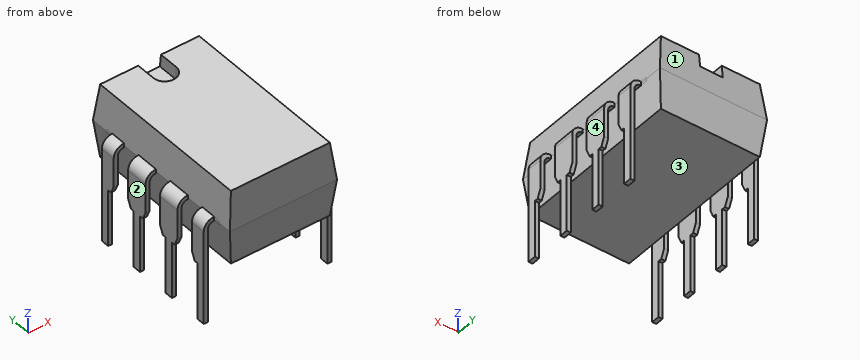
```python
from build123d import *

# Parameters (mm, degrees)
BASIC_SHAPE_DEPTH              = 5.46
SIDE_PROFILE1_DEPTH            = 4.3
SIDE_PROFILE1_DEPTH_BACK       = 4.3
SIDE_PROFILE2_DEPTH            = 4.3
SIDE_PROFILE2_DEPTH_BACK       = 4.3
LOCATION_MARK_DEPTH            = 0.8
SKETCH6_W                      = 0.25
SKETCH6_H                      = 1.39
PIN_RELIEF_DEPTH               = 8.235
REMAINING_PINS_COUNT           = 4
REMAINING_PINS_PITCH           = 2.54
REMAINING_PINS_COPY_1_SKETCH_W = 0.25
REMAINING_PINS_COPY_1_SKETCH_H = 1.39
REMAINING_PINS_COPY_2_SKETCH_W = 0.25
REMAINING_PINS_COPY_2_SKETCH_H = 1.39
REMAINING_PINS_COPY_3_SKETCH_W = 0.25
REMAINING_PINS_COPY_3_SKETCH_H = 1.39
REMAINING_PINS_COPY_4_DEPTH    = 8.235
REMAINING_PINS_COPY_5_DEPTH    = 8.235
REMAINING_PINS_COPY_6_DEPTH    = 8.235
PIN_SHAPE1_DEPTH               = 0.445
PIN_SHAPE2_DEPTH               = 0.445


with BuildPart() as part:
    # Sketch1 → Basic Shape (new body, symmetric)
    with BuildSketch(Plane(origin=(0, 0, 0), x_dir=(1, 0, 0), z_dir=(0, 1, 0))):
        Polygon((-3.05, -0.51), (-3.3, -2.795), (-3.05, -5.08), (3.05, -5.08), (3.3, -2.795), (3.05, -0.51), align=None)
    extrude(amount=BASIC_SHAPE_DEPTH, both=True)

    # Sketch2 → Side Profile1 (cut, two sides)
    with BuildSketch(Plane(origin=(0, 0, 0), x_dir=(0, 0, -1), z_dir=(1, 0, 0))) as side_profile1_sk:
        Polygon((-5.08, 5.46), (-5.08, 5.21), (-2.795, 5.46), align=None)
        Polygon((-5.08, -5.46), (-2.795, -5.46), (-5.08, -5.21), align=None)
    extrude(amount=SIDE_PROFILE1_DEPTH, mode=Mode.SUBTRACT)
    extrude(side_profile1_sk.sketch, amount=-SIDE_PROFILE1_DEPTH_BACK, mode=Mode.SUBTRACT)

    # Sketch3 → Side Profile2 (cut, two sides)
    with BuildSketch(Plane(origin=(0, 0, 0), x_dir=(0, 0, -1), z_dir=(1, 0, 0))) as side_profile2_sk:
        Polygon((-2.795, 5.46), (-0.51, 5.46), (-0.51, 5.21), align=None)
        Polygon((-2.795, -5.46), (-0.51, -5.46), (-0.51, -5.21), align=None)
    extrude(amount=SIDE_PROFILE2_DEPTH, mode=Mode.SUBTRACT)
    extrude(side_profile2_sk.sketch, amount=-SIDE_PROFILE2_DEPTH_BACK, mode=Mode.SUBTRACT)

    # Sketch4 → Location Mark (cut)
    with BuildSketch(Plane(origin=(0, 0, 5.08), x_dir=(-1, 0, 0), z_dir=(0, 0, -1))):
        with BuildLine():
            Line((0.7, 6.21), (-0.7, 6.21))
            Line((-0.7, 6.21), (-0.7, 5.21))
            Line((-0.7, 5.21), (-0.7, 4.01))
            ThreePointArc((-0.7, 4.01), (0, 3.31), (0.7, 4.01))
            Line((0.7, 4.01), (0.7, 5.21))
            Line((0.7, 5.21), (0.7, 6.21))
        make_face()
    extrude(amount=LOCATION_MARK_DEPTH, mode=Mode.SUBTRACT)

    # First Pin: sweep along a path in Sketch5
    with BuildLine(Plane(origin=(0, -3.94, 0), x_dir=(1, 0, 0), z_dir=(0, 1, 0))) as first_pin_path:
        Line((0, -2.795), (3.31, -2.795))
        ThreePointArc((3.31, -2.795), (3.663553391, -2.648553391), (3.81, -2.295))
        Line((3.81, -2.295), (3.81, 3.5))
    # Sketch6 → First Pin (sweep)
    with BuildSketch(Plane(origin=(0, 0, 0), x_dir=(0, 0, -1), z_dir=(1, 0, 0))):
        with Locations((-2.795, -3.94)):
            Rectangle(SKETCH6_W, SKETCH6_H)
    first_pin = sweep(path=first_pin_path.line)

    # Sketch7 → Pin Relief (cut, through all)
    with BuildSketch(Plane(origin=(3.935, 0, 0), x_dir=(0, 0, -1), z_dir=(1, 0, 0))):
        Polygon((0, -4.19), (3.5, -4.19), (3.5, -4.635), (-0.51, -4.635), (0, -4.4125), align=None)
        Polygon((0, -3.69), (3.5, -3.69), (3.5, -3.245), (-0.51, -3.245), (0, -3.4675), align=None)
    pin_relief = extrude(amount=-PIN_RELIEF_DEPTH, mode=Mode.SUBTRACT)

    # Opp Pin: First Pin, Pin Relief across plane
    add(first_pin.mirror(Plane(origin=(0, 0, 0), x_dir=(0, 0, 1), z_dir=(1, 0, 0))))
    add(pin_relief.mirror(Plane(origin=(0, 0, 0), x_dir=(0, 0, 1), z_dir=(1, 0, 0))), mode=Mode.SUBTRACT)

    # Remaining Pins: First Pin, Pin Relief ×4
    with Locations(*[(0, i * REMAINING_PINS_PITCH, 0) for i in range(1, REMAINING_PINS_COUNT)]):
        add(first_pin)
        add(pin_relief, mode=Mode.SUBTRACT)

    # Remaining Pins copy 1: sweep along a path in Remaining Pins copy 1 path
    with BuildLine(Plane(origin=(0, -1.4, 0), x_dir=(-1, 0, 0), z_dir=(0, 1, 0))) as remaining_pins_copy_1_path:
        Line((0, 2.795), (3.31, 2.795))
        ThreePointArc((3.31, 2.795), (3.663553391, 2.648553391), (3.81, 2.295))
        Line((3.81, 2.295), (3.81, -3.5))
    # Remaining Pins copy 1 sketch → Remaining Pins copy 1 (sweep)
    with BuildSketch(Plane(origin=(0, 2.54, 0), x_dir=(0, 0, -1), z_dir=(-1, 0, 0))):
        with Locations((-2.795, 3.94)):
            Rectangle(REMAINING_PINS_COPY_1_SKETCH_W, REMAINING_PINS_COPY_1_SKETCH_H)
    sweep(path=remaining_pins_copy_1_path.line)

    # Remaining Pins copy 2: sweep along a path in Remaining Pins copy 2 path
    with BuildLine(Plane(origin=(0, 1.14, 0), x_dir=(-1, 0, 0), z_dir=(0, 1, 0))) as remaining_pins_copy_2_path:
        Line((0, 2.795), (3.31, 2.795))
        ThreePointArc((3.31, 2.795), (3.663553391, 2.648553391), (3.81, 2.295))
        Line((3.81, 2.295), (3.81, -3.5))
    # Remaining Pins copy 2 sketch → Remaining Pins copy 2 (sweep)
    with BuildSketch(Plane(origin=(0, 5.08, 0), x_dir=(0, 0, -1), z_dir=(-1, 0, 0))):
        with Locations((-2.795, 3.94)):
            Rectangle(REMAINING_PINS_COPY_2_SKETCH_W, REMAINING_PINS_COPY_2_SKETCH_H)
    sweep(path=remaining_pins_copy_2_path.line)

    # Remaining Pins copy 3: sweep along a path in Remaining Pins copy 3 path
    with BuildLine(Plane(origin=(0, 3.68, 0), x_dir=(-1, 0, 0), z_dir=(0, 1, 0))) as remaining_pins_copy_3_path:
        Line((0, 2.795), (3.31, 2.795))
        ThreePointArc((3.31, 2.795), (3.663553391, 2.648553391), (3.81, 2.295))
        Line((3.81, 2.295), (3.81, -3.5))
    # Remaining Pins copy 3 sketch → Remaining Pins copy 3 (sweep)
    with BuildSketch(Plane(origin=(0, 7.62, 0), x_dir=(0, 0, -1), z_dir=(-1, 0, 0))):
        with Locations((-2.795, 3.94)):
            Rectangle(REMAINING_PINS_COPY_3_SKETCH_W, REMAINING_PINS_COPY_3_SKETCH_H)
    sweep(path=remaining_pins_copy_3_path.line)

    # Remaining Pins copy 4 sketch → Remaining Pins copy 4 (cut, through all)
    with BuildSketch(Plane(origin=(-3.935, 2.54, 0), x_dir=(0, 0, -1), z_dir=(-1, 0, 0))):
        Polygon((0, 4.19), (3.5, 4.19), (3.5, 4.635), (-0.51, 4.635), (0, 4.4125), align=None)
        Polygon((0, 3.69), (3.5, 3.69), (3.5, 3.245), (-0.51, 3.245), (0, 3.4675), align=None)
    extrude(amount=-REMAINING_PINS_COPY_4_DEPTH, mode=Mode.SUBTRACT)

    # Remaining Pins copy 5 sketch → Remaining Pins copy 5 (cut, through all)
    with BuildSketch(Plane(origin=(-3.935, 5.08, 0), x_dir=(0, 0, -1), z_dir=(-1, 0, 0))):
        Polygon((0, 4.19), (3.5, 4.19), (3.5, 4.635), (-0.51, 4.635), (0, 4.4125), align=None)
        Polygon((0, 3.69), (3.5, 3.69), (3.5, 3.245), (-0.51, 3.245), (0, 3.4675), align=None)
    extrude(amount=-REMAINING_PINS_COPY_5_DEPTH, mode=Mode.SUBTRACT)

    # Remaining Pins copy 6 sketch → Remaining Pins copy 6 (cut, through all)
    with BuildSketch(Plane(origin=(-3.935, 7.62, 0), x_dir=(0, 0, -1), z_dir=(-1, 0, 0))):
        Polygon((0, 4.19), (3.5, 4.19), (3.5, 4.635), (-0.51, 4.635), (0, 4.4125), align=None)
        Polygon((0, 3.69), (3.5, 3.69), (3.5, 3.245), (-0.51, 3.245), (0, 3.4675), align=None)
    extrude(amount=-REMAINING_PINS_COPY_6_DEPTH, mode=Mode.SUBTRACT)

    # Sketch9 → Pin Shape1 (cut)
    with BuildSketch(Plane.XZ.offset(4.635)):
        with BuildLine():
            Line((3.935, 0), (3.685, 0))
            Line((3.685, 0), (3.685, 2.295))
            ThreePointArc((3.685, 2.295), (3.575165043, 2.560165043), (3.31, 2.67))
            Line((3.31, 2.67), (3.286323851, 2.67))
            Line((3.286323851, 2.67), (3.3, 2.795))
            Line((3.3, 2.795), (3.286323851, 2.92))
            Line((3.286323851, 2.92), (3.31, 2.92))
            ThreePointArc((3.31, 2.92), (3.751941738, 2.736941738), (3.935, 2.295))
            Line((3.935, 2.295), (3.935, 0))
        make_face()
        with BuildLine():
            Line((-3.685, 0), (-3.935, 0))
            Line((-3.935, 0), (-3.935, 2.295))
            ThreePointArc((-3.935, 2.295), (-3.751941738, 2.736941738), (-3.31, 2.92))
            Line((-3.31, 2.92), (-3.286323851, 2.92))
            Line((-3.286323851, 2.92), (-3.3, 2.795))
            Line((-3.3, 2.795), (-3.286323851, 2.67))
            Line((-3.286323851, 2.67), (-3.31, 2.67))
            ThreePointArc((-3.31, 2.67), (-3.575165043, 2.560165043), (-3.685, 2.295))
            Line((-3.685, 2.295), (-3.685, 0))
        make_face()
    extrude(amount=-PIN_SHAPE1_DEPTH, mode=Mode.SUBTRACT)

    # Sketch10 → Pin Shape2 (cut)
    with BuildSketch(Plane(origin=(0, 4.375, 0), x_dir=(-1, 0, 0), z_dir=(0, 1, 0))):
        with BuildLine():
            Line((3.685, 0), (3.935, 0))
            Line((3.935, 0), (3.935, 2.295))
            ThreePointArc((3.935, 2.295), (3.751941738, 2.736941738), (3.31, 2.92))
            Line((3.31, 2.92), (3.286323851, 2.92))
            Line((3.286323851, 2.92), (3.3, 2.795))
            Line((3.3, 2.795), (3.286323851, 2.67))
            Line((3.286323851, 2.67), (3.31, 2.67))
            ThreePointArc((3.31, 2.67), (3.575165043, 2.560165043), (3.685, 2.295))
            Line((3.685, 2.295), (3.685, 0))
        make_face()
        with BuildLine():
            Line((-3.685, 0), (-3.935, 0))
            Line((-3.935, 0), (-3.935, 2.295))
            ThreePointArc((-3.935, 2.295), (-3.751941738, 2.736941738), (-3.31, 2.92))
            Line((-3.31, 2.92), (-3.286323851, 2.92))
            Line((-3.286323851, 2.92), (-3.3, 2.795))
            Line((-3.3, 2.795), (-3.286323851, 2.67))
            Line((-3.286323851, 2.67), (-3.31, 2.67))
            ThreePointArc((-3.31, 2.67), (-3.575165043, 2.560165043), (-3.685, 2.295))
            Line((-3.685, 2.295), (-3.685, 0))
        make_face()
    extrude(amount=-PIN_SHAPE2_DEPTH, mode=Mode.SUBTRACT)


solid = part.part
```
For this review, take the finished solid that the model builds, in its own axes (mm). Face numbers are marked on the shaded views. Coordinates: 2 decimals unless noted, no trailing zeros. Loops run counter-clockwise (first coordinate to the right, second up) from the corner with the lowest first, then second, coordinate; pieces in that order, holes last. Notation, with made-up numbers: (22.25, -28) -> (68.25, -28) arc R14 cw to (68.25, -12) -> close; hole circle Ø8 at (33.25, 20). An arc over 180 degrees is marked (long way). Return JSON: item names as keys, results as strings. Group by question number.
(1) Consider section C-C, the plane y = -0.5. Give the boundary of the cut face in (x, z) (3 decimals), plus the area to 3 significant figures.
(2) To check wall thickness, follow L1, parallel to X at y = 0.75, z = 1.5 (3 decimals); L2, parallel to Z at x = -1.75, y = -0.5; L3, parallel to X at y = -1.75, z = 1.25 (3 decimals). State the ranges of each line that lie inside material, in increasing order.
(3) Mouldability with a two-part tool opening along X and no side actions: class the marked faces 1, 2, 3 and 4 as pulls with the +X half, pulls with the -X half, needs draft (parallel to the pull), parting line crosses it, or undercut.
(4) Consider section B-B, the plane x = 0. Give the boundary of the cut face in (y, z) (3 decimals), plus the area to 3 significant figures.
(5) Consider section A-A, the plane z = -1.5. Count the separate pieces of the cut face and the enclosed holes in it, plus the area to 3 significant figures.
(6) For pin 1 Ø0.5 at (x, z) = (3.5, 1.5) entering from -Y; pin 2 Ø3 at (x, y) = (1.5, -2) entering from -Z; pin 3 Ø2 at (y, z) = (-2, 3.5) entering from +X, all flat-tipped, find the tip position at first contact; note any pin that passes through.
Results below:
{
 "1": {"outline": "(-3.3, 2.795) -> (-3.05, 0.51) -> (3.05, 0.51) -> (3.3, 2.795) -> (3.05, 5.08) -> (-3.05, 5.08) -> close", "area": "29.0 mm2"},
 "2": {"L1": "x = -3.935 to -3.685, -3.158 to 3.158, 3.685 to 3.935", "L2": "z = 0.51 to 5.08", "L3": "x = -3.935 to -3.685, -3.131 to 3.131, 3.685 to 3.935"},
 "3": {"face 1": "needs draft", "face 2": "pulls with the -X half", "face 3": "undercut", "face 4": "pulls with the +X half"},
 "4": {"outline": "(-5.46, 2.795) -> (-5.21, 0.51) -> (5.21, 0.51) -> (5.46, 2.795) -> (5.298, 4.28) -> (3.31, 4.28) -> (3.31, 5.08) -> (-5.21, 5.08) -> close", "area": "47.2 mm2"},
 "5": {"separate pieces": "8", "enclosed holes": "0", "area": "1.00 mm2"},
 "6": {"pin 1": "stops at y = -4.19", "pin 2": "stops at z = 0.51", "pin 3": "stops at x = 3.9"}
}
